Geometry check sheet. Reference: the model listing, model coordinates, mm. Face numbers are marked on the shaded views. A direction names the side the tool comes from. Round coordinates to 2 decimals unless told otherwise and drop trailing zeros. Loops run counter-clockwise (first coordinate to the right, second up) from the corner with the lowest first, then second, coordinate; pieces in that order, holes last.
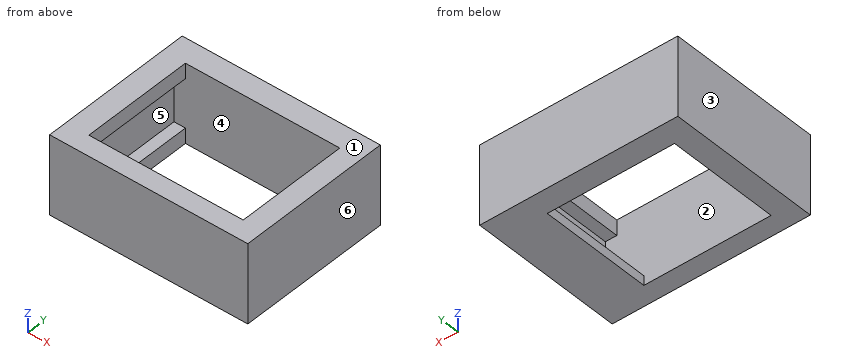
```python
from build123d import *

# Parameters (mm, degrees)
F1_DEPTH = 14.75
F2_DEPTH = 3
F3_W     = 26
F3_H     = 10.4
F4_DEPTH = 2.5
F5_W     = 26
F5_H     = 10.4
F6_DEPTH = 2.5


with BuildPart() as f1:
    # F0 (on Front) → F1 (new body)
    with BuildSketch(Plane.XZ):
        Polygon((3, 10.4), (0, 10.4), (0, 0), (3, 0), (3, 2), (1.5, 2), (1.5, 8.4), (3, 8.4), align=None)
    extrude(amount=F1_DEPTH)



with BuildPart() as f1b:
    # F0 (on Front) → F1, piece 2 (new body)
    with BuildSketch(Plane.XZ):
        Polygon((26, 10.4), (23.25, 10.4), (23.25, 8.4), (24.75, 8.4), (24.75, 5), (19.7, 1.25), (19.7, 0), (26, 0), align=None)
    extrude(amount=F1_DEPTH)


with BuildPart() as f1_1:
    add(f1.part)

    add(f1b.part)  # F2 merges F1b
    # F0 (on Front) → F2 (join)
    with BuildSketch(Plane.XZ):
        Polygon((23.25, 10.4), (3, 10.4), (3, 8.4), (1.5, 8.4), (1.5, 2), (3, 2), (3, 0), (19.7, 0), (19.7, 1.25), (24.75, 5), (24.75, 8.4), (23.25, 8.4), align=None)
        Polygon((26, 10.4), (23.25, 10.4), (23.25, 8.4), (24.75, 8.4), (24.75, 5), (19.7, 1.25), (19.7, 0), (26, 0), align=None)
        Polygon((3, 10.4), (0, 10.4), (0, 0), (3, 0), (3, 2), (1.5, 2), (1.5, 8.4), (3, 8.4), align=None)
    extrude(amount=-F2_DEPTH)

    # F3 (on face) → F4 (join)
    with BuildSketch(Plane.XZ.offset(14.75)):
        with Locations((13, 5.2)):
            Rectangle(F3_W, F3_H)
    extrude(amount=F4_DEPTH)

    # F5 (on Front) → F6 (join)
    with BuildSketch(Plane.XZ):
        with Locations((13, 5.2)):
            Rectangle(F5_W, F5_H)
    extrude(amount=-F6_DEPTH)


solid = f1_1.part
```
1) Sectioned sample at B-B, the plane z = 2.75. Record the cut outline in (x, y).
Report:
outline: (0, -17.25) - (26, -17.25) - (26, 3) - (0, 3) - close; hole (1.5, -14.75) - (21.72, -14.75) - (21.72, 0) - (1.5, 0) - close
2) Sectioned sample at D-D, the plane z = 6.25. Record the cut outline in (x, y).
Report:
outline: (0, -17.25) - (26, -17.25) - (26, 3) - (0, 3) - close; hole (1.5, -14.75) - (24.75, -14.75) - (24.75, 0) - (1.5, 0) - close
3) Access from +Z, -Z, +X, -X, +Y, -Y to the whole of each face (thin tool, end or side, straight path). Record for the marked faces 1 and 2.
Report:
face 1: +Z, +X, -X, +Y, -Y
face 2: none
4) Sectioned sample at C-C, the plane y = -0.5. Record the cut outline in (x, z), then the cut area to 3 significant figures.
Report:
outline: (0, 0) - (3, 0) - (3, 2) - (1.5, 2) - (1.5, 8.4) - (3, 8.4) - (3, 10.4) - (0, 10.4) - close; (19.7, 0) - (26, 0) - (26, 10.4) - (23.25, 10.4) - (23.25, 8.4) - (24.75, 8.4) - (24.75, 5) - (19.7, 1.25) - close
area: 53.4 mm2
5) Mould release check, pull along X, two halves, no side actions. Record for the marked faces 3, 4, 5 and 6: +X half, -X half, draft (parallel to the pull), parting line (faces both ways), or undercut.
Report:
face 3: -X half
face 4: undercut
face 5: undercut
face 6: +X half
6) Scan lines: line 1 along Z through (x, y) = (2.5, -5.5); line 2 along Y through (x, z) = (10.75, 9.25); line 3 along X through (y, z) = (-3, 6.5). Record each from-to range of solid material in increasing order.
Report:
line 1: z = 0 to 2, 8.4 to 10.4
line 2: y = -17.25 to -14.75, 0 to 3
line 3: x = 0 to 1.5, 24.75 to 26
7) Sectioned sample at A-A, the plane x = 14.75. Record the cut outline in (y, z).
Report:
outline: (-17.25, 0) - (-14.75, 0) - (-14.75, 10.4) - (-17.25, 10.4) - close; (0, 0) - (3, 0) - (3, 10.4) - (0, 10.4) - close
